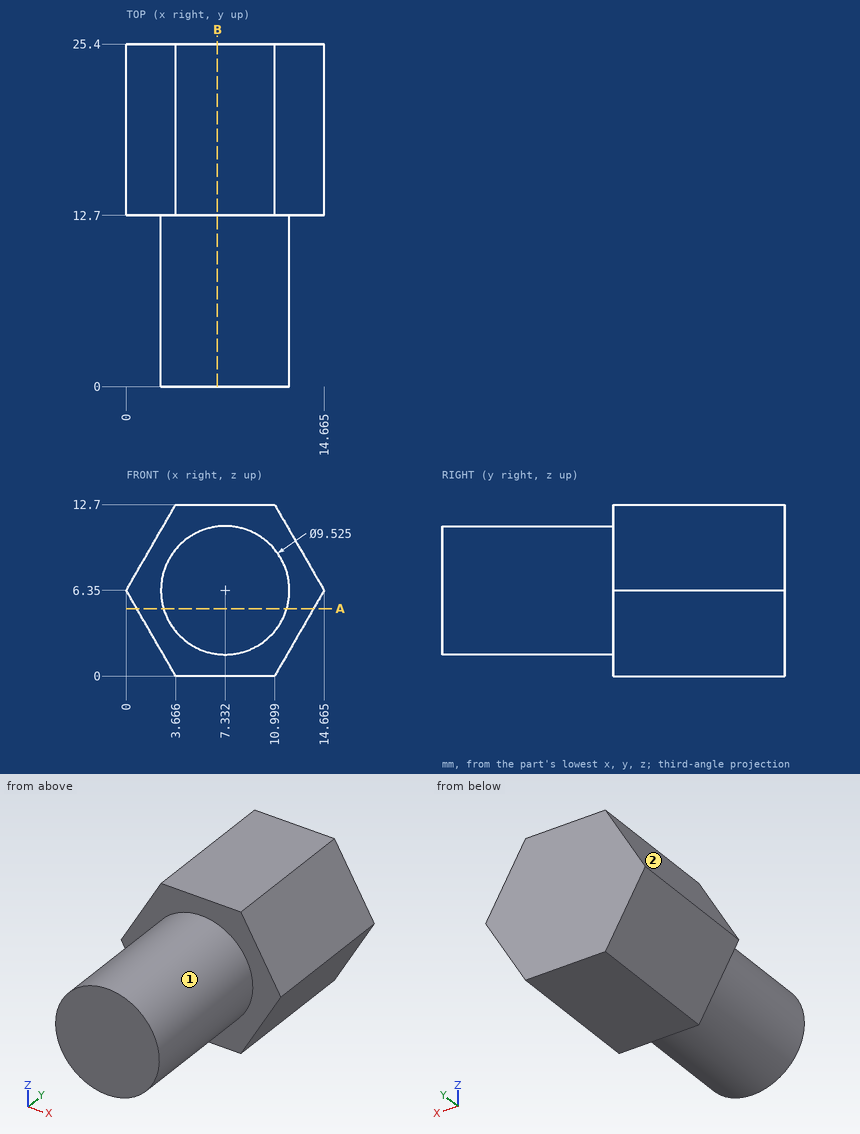
For this review, use the dimensioned drawing (mm, ordinates from the lowest corner) and the shaded views. A direction names the side the tool comes from. Give positions to 0.01 mm unless a question says otherwise; leave off trailing zeros. Order: outer loops, then holes, each group sorted by start corner. A loop starts at its lowest first (then second) coordinate and runs counter-clockwise, first axis right, second up. Notation, with made-up numbers: M 58,56 L 109,56 A33 ccw 109,86 Z; hole C 20,61 d8. An arc over 180 degrees is marked long. Use one line per item in the form item = value. Start each with the question number.
Item 1: We need section A-A on z = 5. Give the boundary of the cut face in (x, y) (1 decimal).
Item 2: To check wall thickness, follow line 1 along Y through (x, z) = (2.25, 3.25); line 2 along X through (y, z) = (12.5, 6.5); line 3 along X through (y, z) = (21.75, 5.75) (1 decimal). State the ranges of each line that lie inside material, in increasing order. Write a range as from..to.
Item 3: We need section B-B on x = 6.75. Give the boundary of the cut face in (y, z).
Item 4: For the marked faces 1 and 2, list the 3-axis set-ups (+Z, -Z, +X, -X, +Y, -Y) from which the entire face can be reached by the end or side of a thin tool; tool diameter is ignored.
Item 5: Insertion check: pin 1 Ø3 at (y, z) = (9.5, 4) entering from -X; pin 2 Ø3 at (x, y) = (2, 17) entering from +Z (1 decimal). Each pin has a flat end and moves straight along its axis. Give the tip position at first contact, or say it passes through.
Completed:
q1.outline = M 0.8,12.7 L 2.8,12.7 L 2.8,0 L 11.9,0 L 11.9,12.7 L 13.9,12.7 L 13.9,25.4 L 0.8,25.4 Z
q2.line_1 = 12.7..25.4
q2.line_2 = 2.57..12.09
q2.line_3 = 0.3..14.3
q3.outline = M 0,1.62 L 12.7,1.62 L 12.7,0 L 25.4,0 L 25.4,12.7 L 12.7,12.7 L 12.7,11.08 L 0,11.08 Z
q4.face_1 = -Y
q4.face_2 = +Z, -X, +Y, -Y
q5.pin_1 = 2.65
q5.pin_2 = 12.4
